Read the model definition and answer for the solid it produces. Units are mm, in the model's axes. A direction names the side the tool comes from. Round coordinates to 2 decimals unless told otherwise and drop trailing zeros. Write each loop counter-clockwise with the first axis right and the second up, starting at its lowest first coordinate (ties: lowest second). Pieces come first, ordered by that corner, then holes. Notation, with made-up numbers: (-40, 18.5) - (-15, 18.5) arc R16 ccw to (-15, 45.5) - close; hole circle Ø3 at (8, 38). An arc over 180 degrees is marked (long way). Use one line per item in the form item = value. Start each with the question number.
1) Consider line 1 along X through (y, z) = (0.75, -29); line 2 along Z through (x, y) = (-13.5, 4.75); line 3 along X through (y, z) = (5, 6.5). Determine where each line is inside the solid, lowest interval first. Write a range as from..to.
2) For a pull along X with two mould halves and no side action, classify faces 4 (the face through (-25.247, 3, 2)), 5 (the face through (-2, 6, 40.471)), 6 (the face through (-7.997, 2, 38)) as released by +X, released by -X, zero draft, split by the parting line, or undercut.
3) The part is cut by section A-A, the plane y = 2.25. Give the vertices of the cut face in (x, z), plus the area to 3 significant figures.
4) The part is cut by section C-C, the plane x = -15. Give the vertices of the cut face in (y, z).
5) The part is cut by section D-D, the plane y = -2. Give the vertices of the cut face in (x, z), plus the area to 3 significant figures.
6) The part is cut by section B-B, the plane z = 33. Give the vertices of the cut face in (x, y), plus the area to 3 significant figures.
7) Each of these flat-tipped pins is pushed along its axis until it touches: pin 1 (8.5 mm diameter, centred on x = -19, z = 13, fed in from -Y); pin 2 (0.9 mm diameter, centred on y = -1.5, z = 28, fed in from +X); pin 3 (2.5 mm diameter, centred on x = -16, y = -2, fed in from +Z). Where does it stop, or does it pass through?
8) For faces 1 (the face through (-23, 7, 2)), 2 (the face through (-20.247, 3, 2)), 3 (the face through (-2, 5, -34)), determine the directions among +Z, -Z, +X, -X, +Y, -Y from which every point of the face is accessible in a straight line to the end or side of a thin tool.
Autodesk Inventor part; units mm, degrees
ref_plane "YZ Plane" through (0, 0, 0) normal (1, 0, 0) x (0, 1, 0)
ref_plane "XZ Plane" through (0, 0, 0) normal (0, 1, 0) x (-1, 0, 0)
ref_plane "XY Plane" through (0, 0, 0) normal (0, 0, 1) x (1, 0, 0)
sketch "Sketch1" plane through (0, 0, 0) normal (0, 1, 0) x (-1, 0, 0)
  line L0 (25.2467, -36.0292) -> (-21.2533, -36.0292)
  line L1 (-4.0033, -36.0292) -> (-4.0033, -31.0292)
  line L2 (-21.2533, -36.0292) -> (-4.0033, -36.0292)
  line L3 (-4.0033, -36.0292) -> (-4.0033, -31.0292)
  line L4 (-4.0033, -31.0292) -> (-16.2533, -31.0292)
  line L5 (-4.0033, -31.0292) -> (-16.2533, -31.0292)
  line L6 (-16.2533, -31.0292) -> (-16.2533, 35.4708)
  line L7 (-16.2533, -31.0292) -> (-16.2533, 35.4708)
  line L8 (-16.2533, 35.4708) -> (-4.0033, 35.4708)
  line L9 (-4.0033, 35.4708) -> (-4.0033, 40.4708)
  line L10 (-21.2533, 40.4708) -> (25.2467, 40.4708)
  line L11 (-21.2533, -36.0292) -> (-21.2533, 40.4708)
  line L12 (-21.2533, 40.4708) -> (-4.0033, 40.4708)
  line L13 (-21.2533, 40.4708) -> (-21.2533, -36.0292)
  line L14 (7.9967, -31.0292) -> (7.9967, -36.0292)
  line L15 (7.9967, -36.0292) -> (25.2467, -36.0292)
  line L16 (25.2467, -36.0292) -> (25.2467, 40.4708)
  line L17 (25.2467, -36.0292) -> (25.2467, 40.4708)
  line L18 (25.2467, 40.4708) -> (7.9967, 40.4708)
  line L19 (7.9967, 40.4708) -> (7.9967, 35.4708)
  line L20 (7.9967, 35.4708) -> (7.9967, 40.4708)
  line L21 (20.2467, -31.0292) -> (7.9967, -31.0292)
  line L22 (7.9967, -36.0292) -> (7.9967, -31.0292)
  line L23 (7.9967, -31.0292) -> (20.2467, -31.0292)
  line L24 (20.2467, 35.4708) -> (20.2467, -31.0292)
  line L25 (20.2467, -31.0292) -> (20.2467, 35.4708)
  line L26 (7.9967, 35.4708) -> (20.2467, 35.4708)
  line L27 (20.2467, 35.4708) -> (7.9967, 35.4708)
  point P0 (0, 0)
extrude "Extrusion1" add sketch "Sketch1" along normal blind 5 contours L0 L14 L21 L24 L26 L19 L10 L16 | L0 L11 L10 L9 L8 L6 L4 L1
sketch "Sketch2" plane through (0, 5, 0) normal (0, 1, 0) x (1, 0, 0)
  point P0 (0, 0)
sketch "Sketch3" plane through (0, 5, 0) normal (0, 1, 0) x (1, 0, 0)
  line L0 (-20.2467, -35.4708) -> (-20.2467, 31.0292)
  line L1 (-20.2467, -35.4708) -> (-10.2467, -35.4708)
  line L2 (-10.2467, -35.4708) -> (-10.2467, -25.4708)
  line L3 (-10.2467, -25.4708) -> (-20.2467, -25.4708)
  line L4 (-20.2467, -25.4708) -> (-20.2467, -35.4708)
  line L5 (16.2533, 31.0292) -> (16.2533, -35.4708)
  line L6 (16.2533, -35.4708) -> (6.2533, -35.4708)
  line L7 (6.2533, -35.4708) -> (6.2533, -25.4708)
  line L8 (6.2533, -25.4708) -> (16.2533, -25.4708)
  line L9 (16.2533, -25.4708) -> (16.2533, -35.4708)
  line L10 (-20.2467, 31.0292) -> (-10.2467, 31.0292)
  line L11 (-10.2467, 31.0292) -> (-10.2467, 21.0292)
  line L12 (-10.2467, 21.0292) -> (-20.2467, 21.0292)
  line L13 (-20.2467, 21.0292) -> (-20.2467, 31.0292)
  point P0 (0, 0)
  dimension "d2" = 10
  dimension "d3" = 10
  dimension "d4" = 10
  dimension "d5" = 10
  dimension "d6" = 10
  dimension "d7" = 10
extrude "Extrusion2" add sketch "Sketch3" against normal blind 8
sketch "Sketch4" plane through (0, 5, 0) normal (0, 1, 0) x (1, 0, 0)
  line L0 (-25.2467, 36.0292) -> (-25.2467, -40.4708)
  line L1 (21.2533, -40.4708) -> (21.2533, 36.0292)
  line L2 (-25.2467, -40.4708) -> (21.2533, -40.4708)
  line L3 (21.2533, -40.4708) -> (21.2533, 36.0292)
  line L4 (21.2533, 36.0292) -> (-25.2467, 36.0292)
  line L5 (-25.2467, 36.0292) -> (-25.2467, -40.4708)
  line L6 (16.2533, 31.0292) -> (16.2533, -25.4708)
  line L7 (-20.2467, -35.4708) -> (-20.2467, -25.4708)
  line L8 (16.2533, 31.0292) -> (-20.2467, 31.0292)
  line L9 (-20.2467, 31.0292) -> (-20.2467, -35.4708)
  line L10 (-20.2467, -35.4708) -> (16.2533, -35.4708)
  line L11 (16.2533, -35.4708) -> (16.2533, 31.0292)
  point P0 (0, 0)
extrude "Extrusion3" add sketch "Sketch4" along normal blind 2
sketch "Sketch5" plane through (0, 5, 0) normal (0, 1, 0) x (1, 0, 0)
  line L0 (-10.2467, -25.4708) -> (-10.2467, -35.4708)
  line L1 (-20.2467, -35.4708) -> (-20.2467, -25.4708)
  line L2 (-10.2467, -25.4708) -> (-20.2467, -25.4708)
  line L3 (-20.2467, -25.4708) -> (-20.2467, -35.4708)
  line L4 (-20.2467, -35.4708) -> (-10.2467, -35.4708)
  line L5 (-10.2467, -35.4708) -> (-10.2467, -25.4708)
  line L6 (-20.2467, 21.0292) -> (-10.2467, 21.0292)
  line L7 (-20.2467, 31.0292) -> (16.2533, 31.0292)
  line L8 (-10.2467, 21.0292) -> (-20.2467, 21.0292)
  line L9 (-20.2467, 21.0292) -> (-20.2467, 31.0292)
  line L10 (-20.2467, 31.0292) -> (-10.2467, 31.0292)
  line L11 (-10.2467, 31.0292) -> (-10.2467, 21.0292)
  line L12 (16.2533, -25.4708) -> (6.2533, -25.4708)
  line L13 (16.2533, -25.4708) -> (16.2533, -35.4708)
  line L14 (6.2533, -25.4708) -> (16.2533, -25.4708)
  line L15 (16.2533, -25.4708) -> (16.2533, -35.4708)
  line L16 (16.2533, -35.4708) -> (6.2533, -35.4708)
  line L17 (6.2533, -35.4708) -> (6.2533, -25.4708)
  point P0 (0, 0)
extrude "Extrusion4" add sketch "Sketch5" along normal blind 2
properties part number "voltage buckboost cover top"
Geometry results:
q1.line_1 = -25.25..-10.25, 16.25..21.25
q1.line_2 = -36.03..-21.03, 25.47..40.47
q1.line_3 = -25.25..-20.25, 16.25..21.25
q2.face_4 = released by -X
q2.face_5 = zero draft
q2.face_6 = undercut
q3.outline = (-25.25, -36.03) - (-8, -36.03) - (-8, -31.03) - (-10.25, -31.03) - (-10.25, -21.03) - (-20.25, -21.03) - (-20.25, 25.47) - (-10.25, 25.47) - (-10.25, 35.47) - (-8, 35.47) - (-8, 40.47) - (-25.25, 40.47) - close; (4, -36.03) - (21.25, -36.03) - (21.25, 40.47) - (4, 40.47) - (4, 35.47) - (6.25, 35.47) - (6.25, 25.47) - (16.25, 25.47) - (16.25, -31.03) - (4, -31.03) - close
q3.area = 1,310 mm2
q4.outline = (-3, -31.03) - (0, -31.03) - (0, -36.03) - (7, -36.03) - (7, -21.03) - (-3, -21.03) - close; (-3, 25.47) - (7, 25.47) - (7, 40.47) - (0, 40.47) - (0, 35.47) - (-3, 35.47) - close
q5.outline = (-20.25, -31.03) - (-10.25, -31.03) - (-10.25, -21.03) - (-20.25, -21.03) - close; (-20.25, 25.47) - (-10.25, 25.47) - (-10.25, 35.47) - (-20.25, 35.47) - close; (6.25, 25.47) - (16.25, 25.47) - (16.25, 35.47) - (6.25, 35.47) - close
q5.area = 300 mm2
q6.outline = (-25.25, 0) - (-20.25, 0) - (-20.25, -3) - (-10.25, -3) - (-10.25, 7) - (-25.25, 7) - close; (6.25, -3) - (16.25, -3) - (16.25, 0) - (21.25, 0) - (21.25, 7) - (6.25, 7) - close
q6.area = 270 mm2
q7.pin_1 = 0
q7.pin_2 = 16.25
q7.pin_3 = 35.47
q8.face_1 = +Z, -Z, +X, -X, +Y
q8.face_2 = +Y, -Y
q8.face_3 = +Z, -Z, -Y
